Check sheet for the modelled part. Datum: model origin and axes. Units: mm. Face numbers are marked on the shaded views. A direction names the side the tool comes from. Round coordinates to 2 decimals unless told otherwise and drop trailing zeros. Use CSV: the item, a comma, the result in double quotes.
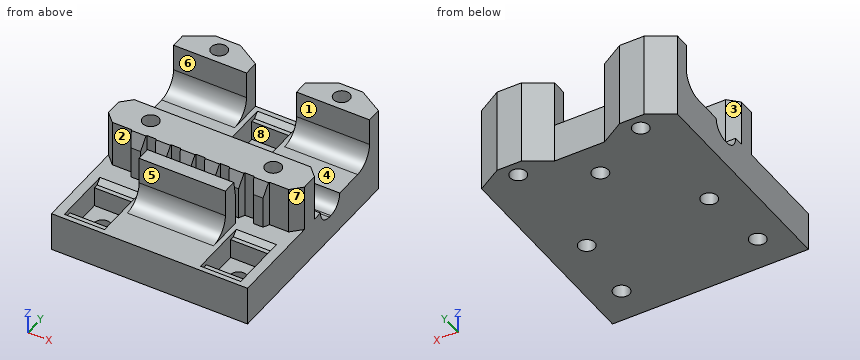
```python
from build123d import *
from OCP.BRepFilletAPI import BRepFilletAPI_MakeChamfer

# Parameters (mm, degrees)
SKETCH1_W                       = 40
SKETCH1_H                       = 44
BOSS_EXTRUDE1_DEPTH             = 8
SKETCH2_W                       = 8.2
SKETCH2_H                       = 10
CUT_EXTRUDE1_DEPTH              = 1
SKETCH3_W                       = 8.2
SKETCH3_H                       = 8.2
CUT_EXTRUDE2_DEPTH              = 4
CHAMFER1_SIZE                   = 1
SKETCH4_R                       = 1.65
CUT_EXTRUDE3_DEPTH              = 56.398555938
SKETCH5_W                       = 17.6
SKETCH5_H                       = 3.325
BOSS_EXTRUDE2_DEPTH             = 9.5
BOSS_EXTRUDE2_DIRECTION_2_REACH = 57.749
FILLET1_R                       = 4
SKETCH6_R                       = 1.65
CUT_EXTRUDE4_DEPTH              = 60.893655758
CHAMFER2_SIZE                   = 2
SKETCH7_W                       = 40
SKETCH7_H                       = 6.5
CUT_EXTRUDE5_DEPTH              = 3
FILLET2_R                       = 3
CHAMFER3_SIZE                   = 3
CHAMFER3_SIZE2                  = 1
CHAMFER4_SIZE                   = 3
CHAMFER4_SIZE2                  = 0.5


with BuildPart() as part:
    # Sketch1 → Boss-Extrude1 (new body)
    with BuildSketch(Plane.XY):
        with Locations((20, 16)):
            Rectangle(SKETCH1_W, SKETCH1_H)
    extrude(amount=BOSS_EXTRUDE1_DEPTH)

    # Sketch2 → Cut-Extrude1 (cut)
    with BuildSketch(Plane.XY.offset(8)):
        with Locations((20, 31)):
            Rectangle(SKETCH2_W, SKETCH2_H)
        with Locations((6.1, 1)):
            Rectangle(SKETCH2_W, SKETCH2_H)
        with Locations((33.9, 1)):
            Rectangle(SKETCH2_W, SKETCH2_H)
    extrude(amount=-CUT_EXTRUDE1_DEPTH, mode=Mode.SUBTRACT)

    # Sketch3 → Cut-Extrude2 (cut)
    with BuildSketch(Plane.XY.offset(7)):
        with Locations((20, 31)):
            Rectangle(SKETCH3_W, SKETCH3_H)
        with Locations((6.1, 1)):
            Rectangle(SKETCH3_W, SKETCH3_H)
        with Locations((33.9, 1)):
            Rectangle(SKETCH3_W, SKETCH3_H)
    extrude(amount=-CUT_EXTRUDE2_DEPTH, mode=Mode.SUBTRACT)

    # Chamfer1
    chamfer1_edges = [part.edges().sort_by_distance(p)[0] for p in [
        (20, 26, 8),
        (20, 36, 8),
        (33.9, -4, 8),
        (33.9, 6, 8),
        (6.1, -4, 8),
        (6.1, 6, 8),
    ]]
    chamfer(chamfer1_edges, length=CHAMFER1_SIZE - 0.0001)  # a hair under: the kernel refuses the full size

    # Sketch4 → Cut-Extrude3 (cut, through all)
    with BuildSketch(Plane.XY.offset(3)):
        with Locations((20, 31)):
            Circle(SKETCH4_R)
        with Locations((6.1, 1)):
            Circle(SKETCH4_R)
        with Locations((33.9, 1)):
            Circle(SKETCH4_R)
    extrude(amount=-CUT_EXTRUDE3_DEPTH, mode=Mode.SUBTRACT)

    # Sketch5 → Boss-Extrude2 (add)
    with BuildSketch(Plane.XY.offset(8)):
        Polygon((20.9, 11.125), (19.1, 11.125), (18.5, 9.925), (16.5, 9.925), (15.9, 11.125), (14.1, 11.125), (13.5, 9.925), (11.5, 9.925), (10.9, 11.125), (9.1, 11.125), (8.5, 9.925), (6.5, 9.925), (5.9, 11.125), (4.1, 11.125), (0, 11.125), (0, 18.5), (40, 18.5), (40, 11.125), (35.9, 11.125), (34.1, 11.125), (33.5, 9.925), (31.5, 9.925), (30.9, 11.125), (29.1, 11.125), (28.5, 9.925), (26.5, 9.925), (25.9, 11.125), (24.1, 11.125), (23.5, 9.925), (21.5, 9.925), align=None)
        with Locations((20, 6.6625)):
            Rectangle(SKETCH5_W, SKETCH5_H)
        Polygon((0, 35), (14.9, 35), (14.9, 38), (10, 41), (5, 41), (0, 38), align=None)
        Polygon((25.1, 38), (30, 41), (35, 41), (40, 38), (40, 35), (25.1, 35), align=None)
    extrude(amount=BOSS_EXTRUDE2_DEPTH)

    # Boss-Extrude2 direction 2: up to this face of the body (flat: up to its plane)
    boss_extrude2_direction_2_end = Plane(part.part.faces().sort_by_distance((20, 16.073973219, 0))[0])
    # Sketch5 → Boss-Extrude2 direction 2 (add, up to the picked face)
    with BuildSketch(Plane.XY.offset(8), mode=Mode.PRIVATE) as boss_extrude2_direction_2_sk1:
        Polygon((20.9, 11.125), (19.1, 11.125), (18.5, 9.925), (16.5, 9.925), (15.9, 11.125), (14.1, 11.125), (13.5, 9.925), (11.5, 9.925), (10.9, 11.125), (9.1, 11.125), (8.5, 9.925), (6.5, 9.925), (5.9, 11.125), (4.1, 11.125), (0, 11.125), (0, 18.5), (40, 18.5), (40, 11.125), (35.9, 11.125), (34.1, 11.125), (33.5, 9.925), (31.5, 9.925), (30.9, 11.125), (29.1, 11.125), (28.5, 9.925), (26.5, 9.925), (25.9, 11.125), (24.1, 11.125), (23.5, 9.925), (21.5, 9.925), align=None)
    boss_extrude2_direction_2_tool1 = split(extrude(boss_extrude2_direction_2_sk1.sketch, amount=-BOSS_EXTRUDE2_DIRECTION_2_REACH, mode=Mode.PRIVATE), bisect_by=boss_extrude2_direction_2_end, keep=Keep.BOTH, mode=Mode.PRIVATE)
    # Sketch5 → Boss-Extrude2 direction 2 (add, up to the picked face)
    with BuildSketch(Plane.XY.offset(8), mode=Mode.PRIVATE) as boss_extrude2_direction_2_sk2:
        with Locations((20, 6.6625)):
            Rectangle(SKETCH5_W, SKETCH5_H)
    boss_extrude2_direction_2_tool2 = split(extrude(boss_extrude2_direction_2_sk2.sketch, amount=-BOSS_EXTRUDE2_DIRECTION_2_REACH, mode=Mode.PRIVATE), bisect_by=boss_extrude2_direction_2_end, keep=Keep.BOTH, mode=Mode.PRIVATE)
    # Sketch5 → Boss-Extrude2 direction 2 (add, up to the picked face)
    with BuildSketch(Plane.XY.offset(8), mode=Mode.PRIVATE) as boss_extrude2_direction_2_sk3:
        Polygon((0, 35), (14.9, 35), (14.9, 38), (10, 41), (5, 41), (0, 38), align=None)
    boss_extrude2_direction_2_tool3 = split(extrude(boss_extrude2_direction_2_sk3.sketch, amount=-BOSS_EXTRUDE2_DIRECTION_2_REACH, mode=Mode.PRIVATE), bisect_by=boss_extrude2_direction_2_end, keep=Keep.BOTH, mode=Mode.PRIVATE)
    # Sketch5 → Boss-Extrude2 direction 2 (add, up to the picked face)
    with BuildSketch(Plane.XY.offset(8), mode=Mode.PRIVATE) as boss_extrude2_direction_2_sk4:
        Polygon((25.1, 38), (30, 41), (35, 41), (40, 38), (40, 35), (25.1, 35), align=None)
    boss_extrude2_direction_2_tool4 = split(extrude(boss_extrude2_direction_2_sk4.sketch, amount=-BOSS_EXTRUDE2_DIRECTION_2_REACH, mode=Mode.PRIVATE), bisect_by=boss_extrude2_direction_2_end, keep=Keep.BOTH, mode=Mode.PRIVATE)
    add(boss_extrude2_direction_2_tool1.solids().sort_by(Axis((20, 14.559414, 8), (0, 0, -1)))[0])
    add(boss_extrude2_direction_2_tool2.solids().sort_by(Axis((20, 6.6625, 8), (0, 0, -1)))[0])
    add(boss_extrude2_direction_2_tool3.solids().sort_by(Axis((7.45835, 37.60161, 8), (0, 0, -1)))[0])
    add(boss_extrude2_direction_2_tool4.solids().sort_by(Axis((32.54165, 37.60161, 8), (0, 0, -1)))[0])

    # Fillet1
    fillet1_edges = [part.edges().sort_by_distance(p)[0] for p in [
        (20, 5, 8),
        (7.45, 35, 8),
        (32.55, 35, 8),
    ]]
    fillet(fillet1_edges, radius=FILLET1_R)

    # Sketch6 → Cut-Extrude4 (cut, through all)
    with BuildSketch(Plane.XY.offset(17.5)):
        with Locations((7.5, 38)):
            Circle(SKETCH6_R)
        with Locations((7.5, 15)):
            Circle(SKETCH6_R)
        with Locations(Location((32.5, 38, 0), (0, 0, 180))):
            Circle(SKETCH6_R)
        with Locations(Location((32.5, 15, 0), (0, 0, 180))):
            Circle(SKETCH6_R)
    extrude(amount=-CUT_EXTRUDE4_DEPTH, mode=Mode.SUBTRACT)

    # Chamfer2
    chamfer2_edges = [part.edges().sort_by_distance(p)[0] for p in [
        (0, 11.125, 12.75),
        (0, 18.5, 12.75),
        (40, 18.5, 12.75),
        (40, 11.125, 12.75),
    ]]
    chamfer(chamfer2_edges, length=CHAMFER2_SIZE)

    # Sketch7 → Cut-Extrude5 (cut)
    with BuildSketch(Plane.XY.offset(8)):
        with Locations((20, 21.75)):
            Rectangle(SKETCH7_W, SKETCH7_H)
    extrude(amount=-CUT_EXTRUDE5_DEPTH, mode=Mode.SUBTRACT)

    # Fillet2
    fillet2_edges = [part.edges().sort_by_distance(p)[0] for p in [
        (20, 18.5, 5),
        (20, 25, 5),
    ]]
    fillet(fillet2_edges, radius=FILLET2_R - 0.0001)  # a hair under: the kernel refuses the full size

    # Chamfer3: one chamfer whose edges measure the first distance from different faces: ONE call of the kernel's chamfer builder (chamfer() names one face for all edges)
    chamfer3_edges_1 = [part.edges().sort_by_distance(p)[0] for p in [
        (22.5, 9.925, 17.5),
    ]]
    chamfer3_side_1 = [part.faces().sort_by_distance(p)[0] for p in [
        (22.5, 9.925, 12.75),
    ]]
    chamfer3_edges_2 = [part.edges().sort_by_distance(p)[0] for p in [
        (27.5, 9.925, 17.5),
    ]]
    chamfer3_side_2 = [part.faces().sort_by_distance(p)[0] for p in [
        (27.5, 9.925, 12.75),
    ]]
    chamfer3_edges_3 = [part.edges().sort_by_distance(p)[0] for p in [
        (32.5, 9.925, 17.5),
    ]]
    chamfer3_side_3 = [part.faces().sort_by_distance(p)[0] for p in [
        (32.5, 9.925, 12.75),
    ]]
    chamfer3_edges_4 = [part.edges().sort_by_distance(p)[0] for p in [
        (7.5, 9.925, 17.5),
    ]]
    chamfer3_side_4 = [part.faces().sort_by_distance(p)[0] for p in [
        (7.5, 9.925, 12.75),
    ]]
    chamfer3_edges_5 = [part.edges().sort_by_distance(p)[0] for p in [
        (12.5, 9.925, 17.5),
    ]]
    chamfer3_side_5 = [part.faces().sort_by_distance(p)[0] for p in [
        (12.5, 9.925, 12.75),
    ]]
    chamfer3_edges_6 = [part.edges().sort_by_distance(p)[0] for p in [
        (17.5, 9.925, 17.5),
    ]]
    chamfer3_side_6 = [part.faces().sort_by_distance(p)[0] for p in [
        (17.5, 9.925, 12.75),
    ]]
    chamfer3 = BRepFilletAPI_MakeChamfer(part.part.solid().wrapped)
    for e in chamfer3_edges_1:
        chamfer3.Add(CHAMFER3_SIZE, CHAMFER3_SIZE2, e.wrapped, chamfer3_side_1[0].wrapped)  # the first distance lies on this face
    for e in chamfer3_edges_2:
        chamfer3.Add(CHAMFER3_SIZE, CHAMFER3_SIZE2, e.wrapped, chamfer3_side_2[0].wrapped)  # the first distance lies on this face
    for e in chamfer3_edges_3:
        chamfer3.Add(CHAMFER3_SIZE, CHAMFER3_SIZE2, e.wrapped, chamfer3_side_3[0].wrapped)  # the first distance lies on this face
    for e in chamfer3_edges_4:
        chamfer3.Add(CHAMFER3_SIZE, CHAMFER3_SIZE2, e.wrapped, chamfer3_side_4[0].wrapped)  # the first distance lies on this face
    for e in chamfer3_edges_5:
        chamfer3.Add(CHAMFER3_SIZE, CHAMFER3_SIZE2, e.wrapped, chamfer3_side_5[0].wrapped)  # the first distance lies on this face
    for e in chamfer3_edges_6:
        chamfer3.Add(CHAMFER3_SIZE, CHAMFER3_SIZE2, e.wrapped, chamfer3_side_6[0].wrapped)  # the first distance lies on this face
    add(Compound.cast(chamfer3.Shape()), mode=Mode.REPLACE)

    # Chamfer4
    chamfer4_edges = [part.edges().sort_by_distance(p)[0] for p in [
        (20, 8.325, 17.5),
    ]]
    chamfer4_side = [part.faces().sort_by_distance(p)[0] for p in [
        (20, 8.325, 12.75),
    ]]
    chamfer(chamfer4_edges, length=CHAMFER4_SIZE, length2=CHAMFER4_SIZE2, reference=chamfer4_side[0])


solid = part.part
```
Q1. Sectioned sample at B-B, the plane z = 9.25. State how many separate pieces and enclosed holes the cut face has, then the cut area to 3 significant figures.
Result sheet:
separate pieces,"4"
enclosed holes,"4"
area,"531 mm^2"
Q2. Access from +Z, -Z, +X, -X, +Y, -Y to the whole of each face (thin tool, end or side, straight path). Record for the marked faces 1, 2, 3, 4 and 5.
Result sheet:
face 1,"+Z, +X, -X"
face 2,"+Z, -X, -Y"
face 3,"+Z, -X"
face 4,"+Z"
face 5,"+Z, +X, -X, -Y"
Q3. Go/stop test with flat-tipped pins: pin 1 (1.2 mm diameter, centred on x = 4, z = 4, fed in from +Y); pin 2 (6.5 mm diameter, centred on x = 27, y = 30.5, fed in from +Z); pin 3 (1.6 mm diameter, centred on x = 28, z = 10, fed in from -Y). Record where each tip stops, or that it passes through.
Result sheet:
pin 1,"stops at y = 40.76"
pin 2,"stops at z = 9.1"
pin 3,"stops at y = 3.86"
Q4. Scan lines: L1, parallel to Y at x = 23, z = 3.25; L2, parallel to Y at x = 20, z = 0.8; L3, parallel to Y at x = 33.9, z = 1.3. Record each from-to range of solid material in increasing order.
Result sheet:
L1,"y = -6 to 26.9, 35.1 to 38"
L2,"y = -6 to 29.35, 32.65 to 38"
L3,"y = -6 to -0.65, 2.65 to 14.13, 15.87 to 37.13, 38.87 to 41"
Q5. Mould release check, pull along X, two halves, no side actions. Record for the marked faces 6, 7 and 8: pulls with the +X half, pulls with the -X half, needs draft (parallel to the pull), parting line crosses it, or undercut.
Result sheet:
face 6,"needs draft"
face 7,"pulls with the +X half"
face 8,"undercut"
